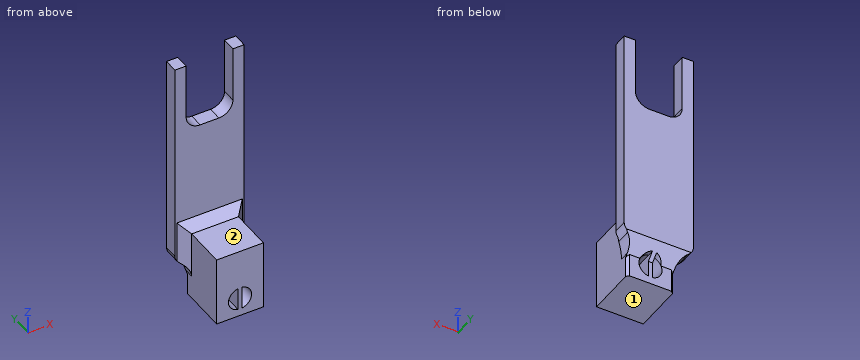
```python
from build123d import *

# Parameters (mm, degrees)
SKETCH1_W           = 12.7
SKETCH1_H           = 19.05
BOSS_EXTRUDE1_DEPTH = 13.97
SKETCH2_W           = 12.7
SKETCH2_H           = 8.89
BOSS_EXTRUDE2_DEPTH = 3.81
CHAMFER3_SIZE       = 3.81
CHAMFER5_SIZE       = 2.54
FILLET1_R           = 3.81
FILLET2_R           = 3.81
FILLET3_R           = 2.54
CHAMFER6_SIZE       = 0.635


with BuildPart() as part:
    # Sketch1 → Boss-Extrude1 (new body)
    with BuildSketch(Plane(origin=(0, 0, 0), x_dir=(1, 0, 0), z_dir=(0, 1, 0))):
        with Locations((6.35, -9.525)):
            Rectangle(SKETCH1_W, SKETCH1_H)
        with BuildLine():
            Line((5.7785, -1.989141169), (5.7785, -8.170858831))
            ThreePointArc((5.7785, -8.170858831), (3.20675, -5.08), (5.7785, -1.989141169))
        make_face(mode=Mode.SUBTRACT)
        with BuildLine():
            ThreePointArc((6.9215, -1.989141169), (9.49325, -5.08), (6.9215, -8.170858831))
            Line((6.9215, -8.170858831), (6.9215, -1.989141169))
        make_face(mode=Mode.SUBTRACT)
    extrude(amount=BOSS_EXTRUDE1_DEPTH)

    # Sketch2 → Boss-Extrude2 (add)
    with BuildSketch(Plane(origin=(0, 13.97, 0), x_dir=(1, 0, 0), z_dir=(0, 1, 0))):
        Polygon((0, -10.16), (-3.048, -10.16), (-3.048, -67.31), (0, -67.31), (0, -48.26), (12.7, -48.26), (12.7, -67.31), (15.748, -67.31), (15.748, -10.16), (12.7, -10.16), (12.7, -19.05), (0, -19.05), align=None)
        with Locations((6.35, -14.605)):
            Rectangle(SKETCH2_W, SKETCH2_H)
    extrude(amount=BOSS_EXTRUDE2_DEPTH)

    # Chamfer3
    # the kernel refuses this chamfer: 3.81 mm, written as the material it adds along each edge
    with BuildSketch(Plane(origin=(12.7, 13.97, 10.16), x_dir=(0, -0.027495876610586382, -0.9996219169112968), z_dir=(-1, 0, 0))) as chamfer3_piece_1_section:
        Polygon((CHAMFER3_SIZE * 0.999621916911, -CHAMFER3_SIZE * 0.0274958766106), (-CHAMFER3_SIZE * 0.0274958766106, -CHAMFER3_SIZE * 0.999621916911), (0, 0), align=None)
    chamfer3_piece_1 = extrude(amount=12.7, mode=Mode.PRIVATE)
    chamfer3_piece_1 = chamfer3_piece_1 - Plane(origin=(6.35, 15.278434863, 5.08), x_dir=(-0.18181818181819312, 0, 0.9833321660356314), z_dir=(0, -1, 0)) * Cylinder(3.14325, 41, mode=Mode.PRIVATE)
    add(chamfer3_piece_1)
    with BuildSketch(Plane(origin=(22.498112184, 13.97, 10.16), x_dir=(0, -0.027495876610586382, -0.9996219169112968), z_dir=(-1, 0, 0))) as chamfer3_piece_2_section:
        Polygon((CHAMFER3_SIZE * 0.999621916911, -CHAMFER3_SIZE * 0.0274958766106), (-CHAMFER3_SIZE * 0.0274958766106, -CHAMFER3_SIZE * 0.999621916911), (0, 0), align=None)
    chamfer3_piece_2 = extrude(amount=32.296224368, mode=Mode.PRIVATE)
    chamfer3_piece_2 = split(chamfer3_piece_2, bisect_by=Plane(origin=(5.7785, 14.588702158, 7.587404322), z_dir=(1, 0, 0)), keep=Keep.TOP, mode=Mode.PRIVATE)
    chamfer3_piece_2 = split(chamfer3_piece_2, bisect_by=Plane(origin=(6.9215, 14.588702158, 7.587404322), z_dir=(-1, 0, 0)), keep=Keep.TOP, mode=Mode.PRIVATE)
    add(chamfer3_piece_2)

    # Chamfer5
    chamfer5_edges = [part.edges().sort_by_distance(p)[0] for p in [
        (6.35, 13.97, 19.05),
        (12.7, 13.97, 14.605),
        (0, 13.97, 14.605),
    ]]
    chamfer(chamfer5_edges, length=CHAMFER5_SIZE)

    # Fillet1
    fillet1_edges = [part.edges().sort_by_distance(p)[0] for p in [
        (0, 15.875, 48.26),
        (12.7, 15.875, 48.26),
    ]]
    fillet(fillet1_edges, radius=FILLET1_R)

    # Fillet2
    # the kernel refuses this fillet: 3.81 mm, written as the material it adds along each edge
    with BuildSketch(Plane(origin=(0, 2.09744408, 10.16), x_dir=(-1.0, 0, -1.5694648846796446e-12), z_dir=(0, 1, 0))) as fillet2_piece_1_section:
        with BuildLine():
            CenterArc((3.81, -3.733022368), FILLET2_R, 101.536959033, 78.463040967)
            Line((0, -3.733022368), (-0.0762, -3.733022368))
            Line((-0.0762, -3.733022368), (-0.0762, 0))
            Line((-0.0762, 0), (0, 0.0762))
            ThreePointArc((0, 0.0762), (1.524, 0.0762), (3.03276, 0.074660447))
            Line((3.03276, 0.074660447), (3.048, 0))
        make_face()
    fillet2_piece_1 = extrude(amount=15.68255592, mode=Mode.PRIVATE)
    fillet2_piece_1 = split(fillet2_piece_1, bisect_by=Plane(origin=(-0.488499052, 13.97, 9.10243743), z_dir=(0, -1, 0)), keep=Keep.TOP, mode=Mode.PRIVATE)
    fillet2_piece_1 = split(fillet2_piece_1, bisect_by=Plane(origin=(-1.001374289, 12.431374289, 9.10243743), z_dir=(0.7071067811865477, 0.7071067811865475, 0)), keep=Keep.TOP, mode=Mode.PRIVATE)
    add(fillet2_piece_1)
    with BuildSketch(Plane(origin=(0, 2.09744408, 10.16), x_dir=(-1.0, 0, -1.5694648846796446e-12), z_dir=(0, 1, 0))) as fillet2_piece_2_section:
        with BuildLine():
            CenterArc((3.81, -3.733022368), FILLET2_R, 101.536959033, 78.463040967)
            Line((0, -3.733022368), (-0.0762, -3.733022368))
            Line((-0.0762, -3.733022368), (-0.0762, 0))
            Line((-0.0762, 0), (0, 0.0762))
            ThreePointArc((0, 0.0762), (1.524, 0.0762), (3.03276, 0.074660447))
            Line((3.03276, 0.074660447), (3.048, 0))
        make_face()
    fillet2_piece_2 = extrude(amount=15.68255592, mode=Mode.PRIVATE)
    fillet2_piece_2 = split(fillet2_piece_2, bisect_by=Plane(origin=(-2.842111613, 13.97, 10.172095318), z_dir=(0, 1, 0)), keep=Keep.TOP, mode=Mode.PRIVATE)
    fillet2_piece_2 = split(fillet2_piece_2, bisect_by=Plane(origin=(-2.766583712, 14.196583712, 10.172095318), z_dir=(-0.7071067811865477, -0.7071067811865475, 0)), keep=Keep.TOP, mode=Mode.PRIVATE)
    add(fillet2_piece_2)
    with BuildSketch(Plane(origin=(0, 2.09744408, 10.16), x_dir=(-1.0, 0, -1.5694648846796446e-12), z_dir=(0, 1, 0))) as fillet2_piece_3_section:
        with BuildLine():
            CenterArc((3.81, -3.733022368), FILLET2_R, 101.536959033, 78.463040967)
            Line((0, -3.733022368), (-0.0762, -3.733022368))
            Line((-0.0762, -3.733022368), (-0.0762, 0))
            Line((-0.0762, 0), (0, 0.0762))
            ThreePointArc((0, 0.0762), (1.524, 0.0762), (3.03276, 0.074660447))
            Line((3.03276, 0.074660447), (3.048, 0))
        make_face()
    fillet2_piece_3 = extrude(amount=15.68255592, mode=Mode.PRIVATE)
    fillet2_piece_3 = split(fillet2_piece_3, bisect_by=Plane(origin=(-0.871394664, 13.97, 9.510267837), z_dir=(0, 1, 0)), keep=Keep.TOP, mode=Mode.PRIVATE)
    fillet2_piece_3 = split(fillet2_piece_3, bisect_by=Plane(origin=(-2.496213957, 13.926213957, 9.510267837), z_dir=(0.7071067811865477, 0.7071067811865475, 0)), keep=Keep.TOP, mode=Mode.PRIVATE)
    fillet2_piece_3 = split(fillet2_piece_3, bisect_by=Plane(origin=(-0.871394664, 16.340650543, 8.720650543), z_dir=(0, -0.7071067811862648, 0.7071067811868302)), keep=Keep.TOP, mode=Mode.PRIVATE)
    add(fillet2_piece_3)
    with BuildSketch(Plane(origin=(12.7, 17.78, 10.16), x_dir=(1.0, 0, -1.0525263949987076e-12), z_dir=(0, -1, 0))) as fillet2_piece_4_section:
        with BuildLine():
            CenterArc((3.81, -3.733022368), FILLET2_R, 101.536959033, 78.463040967)
            Line((0, -3.733022368), (-0.0762, -3.733022368))
            Line((-0.0762, -3.733022368), (-0.0762, 0))
            Line((-0.0762, 0), (0, 0.0762))
            ThreePointArc((0, 0.0762), (1.524, 0.0762), (3.03276, 0.074660447))
            Line((3.03276, 0.074660447), (3.048, 0))
        make_face()
    fillet2_piece_4 = extrude(amount=15.68255592, mode=Mode.PRIVATE)
    fillet2_piece_4 = split(fillet2_piece_4, bisect_by=Plane(origin=(13.571394664, 13.97, 9.510267837), z_dir=(0, 1, 0)), keep=Keep.TOP, mode=Mode.PRIVATE)
    fillet2_piece_4 = split(fillet2_piece_4, bisect_by=Plane(origin=(15.196213957, 13.926213957, 9.510267837), z_dir=(-0.7071067811865479, 0.7071067811865474, 0)), keep=Keep.TOP, mode=Mode.PRIVATE)
    fillet2_piece_4 = split(fillet2_piece_4, bisect_by=Plane(origin=(13.571394664, 16.340650543, 8.720650543), z_dir=(0, -0.7071067811862648, 0.7071067811868302)), keep=Keep.TOP, mode=Mode.PRIVATE)
    add(fillet2_piece_4)
    with BuildSketch(Plane(origin=(12.7, 17.78, 10.16), x_dir=(1.0, 0, -1.0525263949987076e-12), z_dir=(0, -1, 0))) as fillet2_piece_5_section:
        with BuildLine():
            CenterArc((3.81, -3.733022368), FILLET2_R, 101.536959033, 78.463040967)
            Line((0, -3.733022368), (-0.0762, -3.733022368))
            Line((-0.0762, -3.733022368), (-0.0762, 0))
            Line((-0.0762, 0), (0, 0.0762))
            ThreePointArc((0, 0.0762), (1.524, 0.0762), (3.03276, 0.074660447))
            Line((3.03276, 0.074660447), (3.048, 0))
        make_face()
    fillet2_piece_5 = extrude(amount=15.68255592, mode=Mode.PRIVATE)
    fillet2_piece_5 = split(fillet2_piece_5, bisect_by=Plane(origin=(13.188499052, 13.97, 9.10243743), z_dir=(0, -1, 0)), keep=Keep.TOP, mode=Mode.PRIVATE)
    fillet2_piece_5 = split(fillet2_piece_5, bisect_by=Plane(origin=(13.701374289, 12.431374289, 9.10243743), z_dir=(-0.7071067811865479, 0.7071067811865474, 0)), keep=Keep.TOP, mode=Mode.PRIVATE)
    add(fillet2_piece_5)
    with BuildSketch(Plane(origin=(12.7, 17.78, 10.16), x_dir=(1.0, 0, -1.0525263949987076e-12), z_dir=(0, -1, 0))) as fillet2_piece_6_section:
        with BuildLine():
            CenterArc((3.81, -3.733022368), FILLET2_R, 101.536959033, 78.463040967)
            Line((0, -3.733022368), (-0.0762, -3.733022368))
            Line((-0.0762, -3.733022368), (-0.0762, 0))
            Line((-0.0762, 0), (0, 0.0762))
            ThreePointArc((0, 0.0762), (1.524, 0.0762), (3.03276, 0.074660447))
            Line((3.03276, 0.074660447), (3.048, 0))
        make_face()
    fillet2_piece_6 = extrude(amount=15.68255592, mode=Mode.PRIVATE)
    fillet2_piece_6 = split(fillet2_piece_6, bisect_by=Plane(origin=(15.542111613, 13.97, 10.172095318), z_dir=(0, 1, 0)), keep=Keep.TOP, mode=Mode.PRIVATE)
    fillet2_piece_6 = split(fillet2_piece_6, bisect_by=Plane(origin=(15.466583712, 14.196583712, 10.172095318), z_dir=(0.7071067811865479, -0.7071067811865474, 0)), keep=Keep.TOP, mode=Mode.PRIVATE)
    add(fillet2_piece_6)

    # Fillet3
    fillet3_edges = [part.edges().sort_by_distance(p)[0] for p in [
        (-3.048, 15.875, 10.16),
        (15.748, 15.875, 10.16),
    ]]
    fillet(fillet3_edges, radius=FILLET3_R)

    # Chamfer6
    chamfer6_edges = [part.edges().sort_by_distance(p)[0] for p in [
        (12.7, 13.97, 3.175),
        (0, 13.97, 3.175),
    ]]
    chamfer(chamfer6_edges, length=CHAMFER6_SIZE)


solid = part.part
```
The listing builds one solid part. Answer for the finished solid, in the listing's coordinates (mm). Face numbers are marked on the shaded views. A direction names the side the tool comes from. Coordinates: 2 decimals unless noted, no trailing zeros. Loops run counter-clockwise (first coordinate to the right, second up) from the corner with the lowest first, then second, coordinate; pieces in that order, holes last. Notation, with made-up numbers: (74.5, -26.5) - (115.5, -26.5) arc R21 ccw to (115.5, -4.5) - close; hole circle Ø2 at (50, 9.5). An arc over 180 degrees is marked (long way). Use a Markdown table: item, result. Add a question column.
1) The part is cut by section C-C, the plane x = -1. Give the vertices of the cut face in (y, z).
2) Find the intervals of material crossed by line 1 (X direction, y = 2.5, z = 7.5); line 2 (Z direction, x = 10.5, y = 2.5); line 3 (X direction, y = 4.75, z = 6), in increasing order.
3) For the marked faces 1 and 2, determine the directions among +Z, -Z, +X, -X, +Y, -Y from which every point of the face is accessible in a straight line to the end or side of a thin tool.
4) The part is cut by section D-D, the plane z = 45. Give the vertices of the cut face in (x, y), and give its area (3 significant figures).
5) The part is cut by section B-B, the plane x = 7.5. Give the vertices of the cut face in (y, z), and give its area (3 significant figures).
6) The part is cut by section A-A, the plane y = 3. Give the vertices of the cut face in (x, z), and give its area (3 significant figures).
7) Given pin 1 (5 mm diameter, centred on y = 13, z = 34, fed in from -X); pin 2 (3 mm diameter, centred on x = 5, z = 4.5, fed in from +Y); pin 3 (1.9 mm diameter, centred on x = 6, y = 16, fed in from +Z); pin 4 (5 mm diameter, centred on y = 11, z = 6.5, fed in from +X), each flat-ended and moving along its own axis, determine where each tip first touches the part or whether it passes through.
Here are the results:
| question | item | result |
|---|---|---|
| 1 | outline | (12.43, 9) - (16.62, 9) - (17.78, 10.16) - (17.78, 67.31) - (13.97, 67.31) - (13.97, 21.59) - (12.43, 20.05) - close |
| 2 | line 1 | x = 0 to 4.34, 5.78 to 6.92, 8.36 to 12.7 |
| 2 | line 2 | z = 0 to 19.05 |
| 2 | line 3 | x = 0 to 3.34, 5.78 to 6.92, 9.36 to 12.7 |
| 3 | face 1 | -Z, +X, -X, +Y, -Y |
| 3 | face 2 | +Z, +X, -X, -Y |
| 4 | outline | (-3.05, 13.97) - (15.75, 13.97) - (15.75, 17.78) - (-3.05, 17.78) - close |
| 4 | area | 71.6 mm^2 |
| 5 | outline | (0, 0) - (13.97, 0) - (13.97, 2.15) - (0, 2.15) - close; (0, 8.01) - (15.63, 8.01) - (17.78, 10.16) - (17.78, 48.26) - (13.97, 48.26) - (13.97, 21.59) - (11.43, 19.05) - (0, 19.05) - close |
| 5 | area | 339 mm^2 |
| 6 | outline | (0, 0) - (12.7, 0) - (12.7, 19.05) - (0, 19.05) - close; hole (5.78, 1.99) - (5.78, 8.17) arc R3.14 ccw to start; hole (6.92, 1.99) arc R3.14 ccw to (6.92, 8.17) - close |
| 6 | area | 218 mm^2 |
| 7 | pin 1 | stops at x = -3.05 |
| 7 | pin 2 | stops at y = 13.97 |
| 7 | pin 3 | stops at z = 48.26 |
| 7 | pin 4 | stops at x = 13.45 |
